Geometry check sheet. Reference: the model listing, model coordinates, mm. Face numbers are marked on the shaded views. Round coordinates to 2 decimals unless told otherwise and drop trailing zeros. Loops run counter-clockwise (first coordinate to the right, second up) from the corner with the lowest first, then second, coordinate; pieces in that order, holes last.
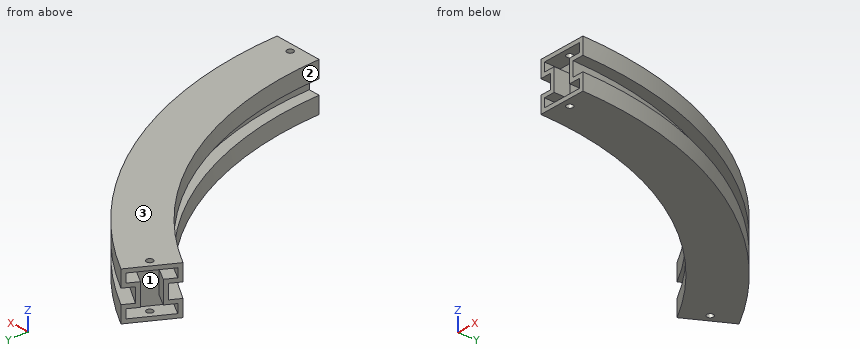
Autodesk Inventor part; units mm, degrees
ref_plane "YZ Plane" through (0, 0, 0) normal (1, 0, 0) x (0, 1, 0)
ref_plane "XZ Plane" through (0, 0, 0) normal (0, 1, 0) x (-1, 0, 0)
ref_plane "XY Plane" through (0, 0, 0) normal (0, 0, 1) x (1, 0, 0)
sketch "Sketch2" plane through (0, 0, 0) normal (0, 1, 0) x (-1, 0, 0)
  line L0 (15, 15) -> (-15, 15)
  line L1 (-15, -15) -> (15, -15)
  line L2 (15, 4.5) -> (8, 4.5)
  line L3 (8, 4.5) -> (8, -4.5)
  line L4 (8, -4.5) -> (15, -4.5)
  line L5 (-15, 4.5) -> (-8, 4.5)
  line L6 (-8, 4.5) -> (-8, -4.5)
  line L7 (-8, -4.5) -> (-15, -4.5)
  line L8 (15, -15) -> (15, -4.5)
  line L9 (15, 4.5) -> (15, 15)
  line L10 (-15, 15) -> (-15, 4.5)
  line L11 (-15, -4.5) -> (-15, -15)
  point P0 (0, 0)
  dimension "d18" = 9
  dimension "d19" = 7
  dimension "d21" = 16
  dimension "d22" = 30
  dimension "d23" = 15
  dimension "d24" = 4.5
  dimension "d25" = 8
sketch "Sketch6" plane through (0, 0, 0) normal (0, 0, 1) x (1, 0, 0)
  arc A0 (0, 0) -> (-110, 190.5256) centre (-220, 0) ccw
  line L0 (-220, 0) -> (-110, 190.5256) construction
  line L1 (-220, 0) -> (0, 0) construction
  dimension "d41" = 220
  dimension "d42" = 60
  dimension "d43" = 220
  dimension "d44" = 0
sweep "Sweep2" add profiles "Sketch2" path "Sketch6"
sketch "Sketch7" plane through (-102.5, 203.516, 4.5) normal (-0.8660254, 0.5, 0) x (0, 0, 1)
  line L0 (-17, -2.5) -> (-11.5, -2.5)
  line L1 (-11.5, -2.5) -> (-11.5, -9.5)
  line L2 (-11.5, -9.5) -> (2.5, -9.5)
  line L3 (2.5, -9.5) -> (2.5, -2.5)
  line L4 (2.5, -2.5) -> (8, -2.5)
  line L5 (8, -2.5) -> (8, -27.5)
  line L6 (8, -27.5) -> (2.5, -27.5)
  line L7 (2.5, -27.5) -> (2.5, -20.5)
  line L8 (2.5, -20.5) -> (-11.5, -20.5)
  line L9 (-11.5, -20.5) -> (-11.5, -27.5)
  line L10 (-11.5, -27.5) -> (-17, -27.5)
  line L11 (-17, -27.5) -> (-17, -2.5)
  line L12 (-19.5, 0) -> (-19.5, -30)
  line L13 (-9, -7) -> (-9, 0)
  line L14 (0, 0) -> (0, -7)
  line L15 (10.5, -30) -> (10.5, 0)
  line L16 (-19.5, -30) -> (-9, -30)
  line L17 (-9, 0) -> (-19.5, 0)
  line L18 (0, -30) -> (10.5, -30)
  line L19 (-9, -23) -> (0, -23)
  line L20 (0, -7) -> (-9, -7)
  point P0 (-4.5, -125)
  point P1 (-14.25, 0)
  dimension "d47" = 2.5
  dimension "d48" = 2.5
  dimension "d49" = 2.5
  dimension "d50" = 2.5
  dimension "d51" = 2.5
  dimension "d52" = 2.5
  dimension "d53" = 2.5
  dimension "d54" = 2.5
  dimension "d55" = 2.5
extrude "Extrusion3" cut sketch "Sketch7" against normal blind 10
sketch "Sketch9" plane through (-15, 0, 15) normal (0, 0, 1) x (1, 0, 0)
  circle A0 centre (-90.6699, 188.0256) radius 2
  line L0 (-90.6699, 188.0256) -> (-95, 190.5256) construction
  line L1 (-95, 190.5256) -> (-102.5, 177.5352) construction
  line L2 (-102.5, 177.5352) -> (-87.5, 203.516)
  point P0 (15, 0)
  dimension "d63" = 4
  dimension "d65" = 5
  dimension "d66" = 15
extrude "Extrusion5" cut sketch "Sketch9" against normal through all
sketch "Sketch10" plane through (-15, 0, 15) normal (0, -1, 0) x (1, 0, 0)
  line L0 (2.5, -2.5) -> (27.5, -2.5)
  line L1 (27.5, -2.5) -> (27.5, -8)
  line L2 (27.5, -8) -> (20.5, -8)
  line L3 (20.5, -8) -> (20.5, -22)
  line L4 (20.5, -22) -> (27.5, -22)
  line L5 (27.5, -22) -> (27.5, -27.5)
  line L6 (27.5, -27.5) -> (2.5, -27.5)
  line L7 (2.5, -27.5) -> (2.5, -22)
  line L8 (2.5, -22) -> (9.5, -22)
  line L9 (9.5, -22) -> (9.5, -8)
  line L10 (9.5, -8) -> (2.5, -8)
  line L11 (2.5, -2.5) -> (2.5, -8)
  line L12 (0, -10.5) -> (0, 0)
  line L13 (0, 0) -> (30, 0)
  line L14 (30, 0) -> (30, -10.5)
  line L15 (7, -19.5) -> (7, -10.5)
  line L16 (23, -10.5) -> (23, -19.5)
  line L17 (30, -30) -> (0, -30)
  line L18 (23, -19.5) -> (30, -19.5)
  line L19 (30, -10.5) -> (23, -10.5)
  point P0 (15, -15)
  point P1 (0, -5.25)
  point P2 (30, -5.25)
  point P3 (23, -15)
  point P4 (26.5, -19.5)
  dimension "d69" = 2.5
  dimension "d70" = 2.5
  dimension "d71" = 2.5
  dimension "d72" = 2.5
  dimension "d73" = 2.5
  dimension "d74" = 2.5
  dimension "d75" = 2.5
  dimension "d76" = 2.5
extrude "Extrusion6" cut sketch "Sketch10" against normal blind 10
sketch "Sketch11" plane through (15, 0, -15) normal (0, 0, -1) x (-1, 0, 0)
  circle A0 centre (15, 5) radius 2
  line L0 (0, 0) -> (30, 0)
  point P0 (15, 0)
  point P1 (15, 0)
  dimension "d79" = 4
  dimension "d80" = 5
  dimension "d81" = 15
extrude "Extrusion7" cut sketch "Sketch11" against normal through all
sketch "Sketch12" plane through (-15, 0, 15) normal (0, 0, 1) x (1, 0, 0)
  line L0 (52.0574, -18.6424) -> (-62.9426, -18.6424)
  line L1 (-62.9426, 220.5256) -> (52.0574, 220.5256)
  line L2 (52.0574, 220.5256) -> (52.0574, -18.6424)
  line L3 (0, 0) -> (30, 0)
  line L4 (-62.9426, 220.5256) -> (-96.15, 163.0087)
  line L5 (-96.15, 163.0087) -> (-96.15, -18.6424)
  line L6 (-62.9426, -18.6424) -> (-96.15, -18.6424)
  line L7 (-102.5, 177.5352) -> (-87.5, 203.516)
  point P0 (15, 0)
  point P1 (15, 0)
  point P2 (15, 0)
  dimension "d85" = 239.168
  dimension "d86" = 37.0574
  dimension "d87" = 18.6424
  dimension "d90" = 148.2074
  dimension "d91" = 115
  dimension "d92" = 181.6511
extrude "Extrusion8" [suppressed]
properties part number "LightRail_endSection"
1) Scan lines: line 1 along Z through (x, y) = (-98, 193); line 2 along Z through (x, y) = (-70.5, 178.5); line 3 along X through (y, z) = (87.5, 9.5). Record each from-to range of solid material in increasing order.
Report:
line 1: z = -15 to -12.5, -7 to -4.5, 4.5 to 7, 12.5 to 15
line 2: z = -15 to -4.5, 4.5 to 15
line 3: x = -34.61 to -1.9
2) Mould release check, pull along Z, two halves, no side actions. Record for the marked faces 1, 2 and 3: +Z half, -Z half, draft (parallel to the pull), parting line (faces both ways), or undercut.
Report:
face 1: undercut
face 2: draft
face 3: +Z half
3) Sectioned sample at B-B, the plane x = 0. Record the cut outline in (y, z), then the cut area to 3 significant figures.
Report:
outline: (0, -15) - (3, -15) - (3, -12.5) - (0, -12.5) - close; (0, 12.5) - (3, 12.5) - (3, 15) - (0, 15) - close; (7, -15) - (82.61, -15) - (82.61, -4.5) - (59.87, -4.5) - (59.87, 4.5) - (82.61, 4.5) - (82.61, 15) - (7, 15) - (7, 12.5) - (10, 12.5) - (10, -12.5) - (7, -12.5) - close
area: 2,000 mm2
4) Sectioned sample at C-C, the plane x = -57. Record the cut outline in (y, z).
Report:
outline: (124.32, -15) - (169.28, -15) - (169.28, -4.5) - (159.42, -4.5) - (159.42, 4.5) - (169.28, 4.5) - (169.28, 15) - (124.32, 15) - (124.32, 4.5) - (135.55, 4.5) - (135.55, -4.5) - (124.32, -4.5) - close
5) Sectioned sample at D-D, the plane y = 59. Record the cut outline in (x, z), then the cut area to 3 significant figures.
Report:
outline: (-23.67, -15) - (7.47, -15) - (7.47, -4.5) - (0.23, -4.5) - (0.23, 4.5) - (7.47, 4.5) - (7.47, 15) - (-23.67, 15) - (-23.67, 4.5) - (-16.38, 4.5) - (-16.38, -4.5) - (-23.67, -4.5) - close
area: 804 mm2
6) Gauge pin test, flat ends, axial feed: pin 1 (5 mm diameter, centred on x = -105.67, y = 188.03, fed in from +Z); pin 2 (1 mm diameter, centred on y = 150.5, z = 7.5, fed in from -X); pin 3 (3 mm diameter, centred on y = 3, z = 2.5, fed in from -X); pin 4 (1 mm diameter, centred on y = 30.5, z = 2.5, fed in from -X). Record the tip position at first contact, or that the pin passes through.
Report:
pin 1: stops at z = 15
pin 2: stops at x = -81.35
pin 3: stops at x = -8.05
pin 4: stops at x = -10.28
